```python
from build123d import *

# Parameters (mm, degrees)
BOSS_EXTRUDE2_DEPTH = 1.524


with BuildPart() as part:
    # Sketch1 → Boss-Extrude2 (new body)
    with BuildSketch(Plane.XY):
        with BuildLine():
            Line((-0.765410013, -0.503143286), (-0.764991894, 2.492240818))
            Line((-0.764991894, 2.492240818), (0.760988125, 2.492240818))
            Line((0.760988125, 2.492240818), (0.760988125, -0.503092163))
            ThreePointArc((0.760988125, -0.503092163), (2.573737831, -1.346888202), (3.55195433, -3.090776309))
            ThreePointArc((3.55195433, -3.090776309), (3.695640119, -6.618686281), (2.730705837, -10.015110313))
            ThreePointArc((2.730705837, -10.015110313), (2.653965632, -11.591332876), (3.221955388, -13.063662413))
            ThreePointArc((3.221955388, -13.063662413), (3.485746852, -11.851447246), (4.275671769, -10.894854243))
            ThreePointArc((4.275671769, -10.894854243), (5.603621463, -8.626073328), (6.594544537, -6.191142388))
            ThreePointArc((6.594544537, -6.191142388), (7.545888132, -4.512710917), (8.849839361, -3.090776309))
            ThreePointArc((8.849839361, -3.090776309), (8.093123436, -3.392493185), (7.283276893, -3.30417195))
            ThreePointArc((7.283276893, -3.30417195), (7.407565604, -2.328155091), (7.47948144, -1.346888202))
            ThreePointArc((7.47948144, -1.346888202), (7.974772805, 1.073186615), (8.849839361, 3.383237301))
            ThreePointArc((8.849839361, 3.383237301), (8.055674116, 2.944556231), (7.154590571, 3.050329405))
            ThreePointArc((7.154590571, 3.050329405), (6.853539824, 4.337001735), (6.46088015, 5.598736896))
            ThreePointArc((6.46088015, 5.598736896), (6.307858777, 6.794433229), (6.46088015, 7.990129562))
            ThreePointArc((6.46088015, 7.990129562), (6.094168188, 7.687528271), (5.630106714, 7.584125409))
            ThreePointArc((5.630106714, 7.584125409), (5.398611626, 7.957700377), (5.106185913, 8.285778776))
            ThreePointArc((5.106185913, 8.285778776), (2.209855231, 11.5967516), (-0.002002475, 15.39924525))
            ThreePointArc((-0.002002475, 15.39924525), (-2.213860181, 11.5967516), (-5.110190864, 8.285778776))
            ThreePointArc((-5.110190864, 8.285778776), (-5.402616576, 7.957700377), (-5.634111665, 7.584125409))
            ThreePointArc((-5.634111665, 7.584125409), (-6.098173139, 7.687528271), (-6.4648851, 7.990129562))
            ThreePointArc((-6.4648851, 7.990129562), (-6.311863727, 6.794433229), (-6.4648851, 5.598736896))
            ThreePointArc((-6.4648851, 5.598736896), (-6.857544775, 4.337001735), (-7.158595522, 3.050329405))
            ThreePointArc((-7.158595522, 3.050329405), (-8.059679066, 2.944556231), (-8.853844312, 3.383237301))
            ThreePointArc((-8.853844312, 3.383237301), (-7.978777755, 1.073186615), (-7.48348639, -1.346888202))
            ThreePointArc((-7.48348639, -1.346888202), (-7.411570554, -2.328155091), (-7.287281843, -3.30417195))
            ThreePointArc((-7.287281843, -3.30417195), (-8.097128387, -3.392493185), (-8.853844312, -3.090776309))
            ThreePointArc((-8.853844312, -3.090776309), (-7.549893082, -4.512710917), (-6.598549488, -6.191142388))
            ThreePointArc((-6.598549488, -6.191142388), (-5.607626413, -8.626073328), (-4.27967672, -10.894854243))
            ThreePointArc((-4.27967672, -10.894854243), (-3.489751802, -11.851447246), (-3.225960338, -13.063662413))
            ThreePointArc((-3.225960338, -13.063662413), (-2.657970582, -11.591332876), (-2.734710788, -10.015110313))
            ThreePointArc((-2.734710788, -10.015110313), (-3.69964507, -6.618686281), (-3.555959281, -3.090776309))
            ThreePointArc((-3.555959281, -3.090776309), (-2.577896844, -1.347030777), (-0.765410013, -0.503143286))
        make_face()
    extrude(amount=BOSS_EXTRUDE2_DEPTH)


solid = part.part
```
For this review, take the finished solid that the model builds, in its own axes (mm). A direction names the side the tool comes from. Give positions to 0.01 mm unless a question says otherwise; leave off trailing zeros. Order: outer loops, then holes, each group sorted by start corner. A loop starts at its lowest first (then second) coordinate and runs counter-clockwise, first axis right, second up.
1) Take a section at C-C (x = 2). Give the boundary of the cut face in (y, z).
2) Take a section at B-B (y = 10). Give the boundary of the cut face in (x, z).
3) Insertion check: pin 1 (0.8 mm diameter, centred on x = 0, z = 1, fed in from -Y). The pin has a flat end and moves straight along its axis. Give the tip position at first contact, or say it passes through.
4) The part is to be moulded in two halves that separate along Y. For faces 5 (the face through (2, 1, 0)), 6 (the face through (-8.047, 2.942, 0.751)), 7 (the face through (-2.6, -1.37, 0.75)), 8 (the face through (3.7, -6.57, 0.75)), say which applies: released by +Y, released by -Y, zero draft, split by the parting line, or undercut.
5) Wall thickness on line 1 (X direction, y = 6.75, z = 0.9); line 2 (X direction, y = -7.5, z = 1.25); line 3 (X direction, y = 7.75, z = 1.45) (3 decimals): over which ranges is each line inside the solid? List them lowest first.
6) For faces 1 (the face through (-6.092, 7.685, 0.751)), 2 (the face through (7.965, 1.04, 0.751)), 3 (the face through (-7.99, 1.11, 0.75)), 4 (the face through (0, 2.492, 1)), list the 3-axis set-ups (+Z, -Z, +X, -X, +Y, -Y) from which the entire face can be reached by the end or side of a thin tool; tool diameter is ignored.
Derived:
1. outline: (-0.92, 0) - (11.89, 0) - (11.89, 1.52) - (-0.92, 1.52) - close
2. outline: (-3.47, 0) - (3.47, 0) - (3.47, 1.52) - (-3.47, 1.52) - close
3. pin 1: stops at y = 2.49
4. face 5: zero draft
4. face 6: released by +Y
4. face 7: undercut
4. face 8: undercut
5. line 1: x = -6.31 to 6.31
5. line 2: x = -6.12 to -3.56, 3.56 to 6.11
5. line 3: x = -6.409 to -6.208, -5.542 to 5.538, 6.204 to 6.405
6. face 1: +Z, -Z, +Y
6. face 2: +Z, -Z, +X
6. face 3: +Z, -Z, -X
6. face 4: +Z, -Z, -Y
